Check sheet for the drawn part. Datum: minimum x, y, z corner. Units: mm. Give positions to 0.01 mm unless a question says otherwise; leave off trailing zeros. Order: outer loops, then holes, each group sorted by start corner. A loop starts at its lowest first (then second) coordinate and runs counter-clockwise, first axis right, second up. Notation, with made-up numbers: (39, 55.5) -> (71, 55.5) arc R14 cw to (71, 60.5) -> close; hole circle Ø11 at (-34, 6). An arc over 180 degrees is marked (long way). Return JSON: item names as keys, results as strings. Group by question number.
(1) Cross-section at A-A on z = 6. Enter the section's corners in (x, y), then the cut area to 3 significant figures.
(2) Cross-section at B-B on x = 6. Enter the section's corners in (y, z).
(3) Thickness scan on line 1 along Z through (x, y) = (6, 3.8); line 2 along X through (y, z) = (1.95, 4.5); line 3 along Z through (x, y) = (2, 1.2). Record the ranges inside material, lowest first.
(4) Release check for a two-part mould opening along Z. For the marked faces 1, 2 and 3 record: pulls with the +Z half, pulls with the -Z half, needs draft (parallel to the pull), parting line crosses it, or undercut.
(5) Cross-section at C-C on y = 1.7. Enter the section's corners in (x, z), then the cut area to 3 significant figures.
(6) Depth check by flat-ended pin: pin 1 Ø1 at (y, z) = (0.5, 1.5) entering from +X; pin 2 Ø3.5 at (x, z) = (6, 6) entering from -Y; pin 3 Ø1 at (x, y) = (5.5, 1.5) entering from -Z; pin 4 Ø2 at (y, z) = (4.5, 10.5) entering from +X. Enter the tip coordinate at first touch or a pass-through.
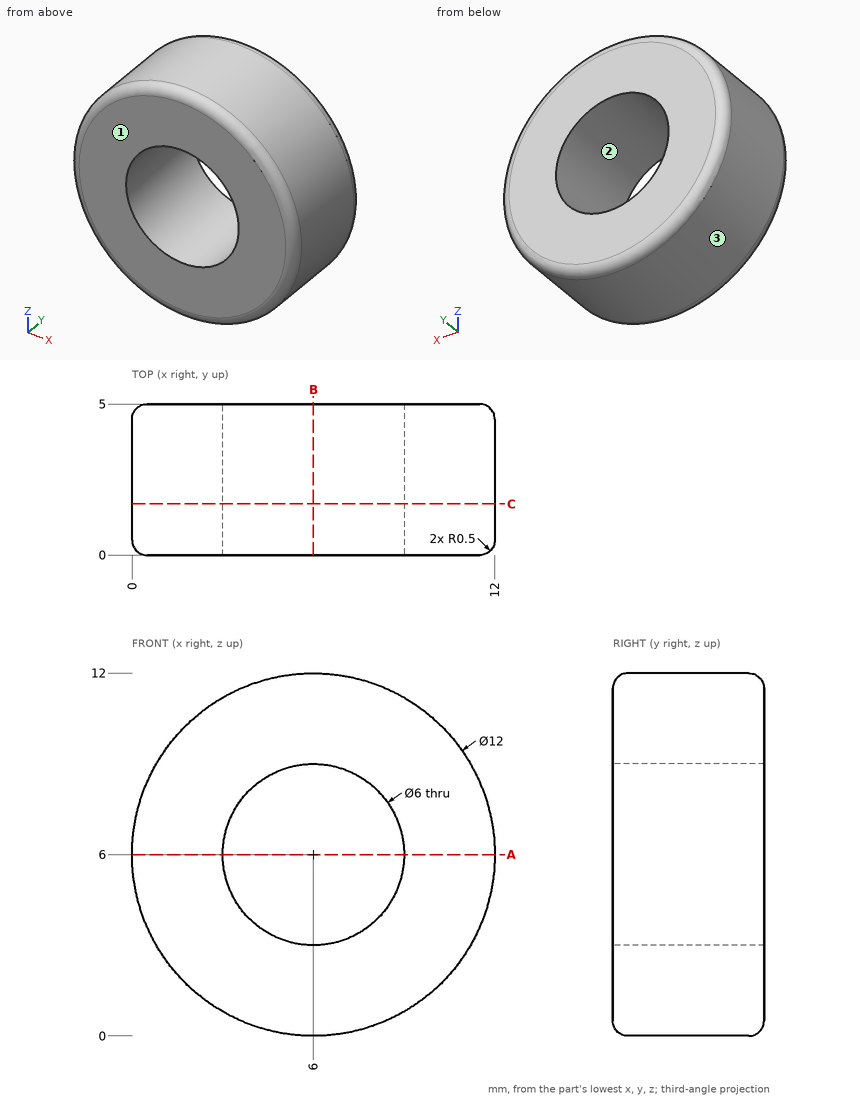
Verdict:
{
 "1": {"outline": "(0, 0.5) arc R0.5 ccw to (0.5, 0) -> (3, 0) -> (3, 5) -> (0.5, 5) arc R0.5 ccw to (0, 4.5) -> close; (9, 0) -> (11.5, 0) arc R0.5 ccw to (12, 0.5) -> (12, 4.5) arc R0.5 ccw to (11.5, 5) -> (9, 5) -> close", "area": "29.8 mm²"},
 "2": {"outline": "(0, 0.5) arc R0.5 ccw to (0.5, 0) -> (4.5, 0) arc R0.5 ccw to (5, 0.5) -> (5, 3) -> (0, 3) -> close; (0, 9) -> (5, 9) -> (5, 11.5) arc R0.5 ccw to (4.5, 12) -> (0.5, 12) arc R0.5 ccw to (0, 11.5) -> close"},
 "3": {"line 1": "0 to 3, 9 to 12", "line 2": "0.19 to 3.4, 8.6 to 11.81", "line 3": "1.53 to 10.47"},
 "4": {"face 1": "needs draft", "face 2": "undercut", "face 3": "parting line crosses it"},
 "5": {"outline": "circle Ø12 at (6, 6); hole circle Ø6 at (6, 6)", "area": "84.8 mm²"},
 "6": {"pin 1": "x = 10.47", "pin 2": "through", "pin 3": "z = 0", "pin 4": "x = 10.87"}
}
